For this review, take the finished solid that the model builds, in its own axes (mm). A direction names the side the tool comes from. Give positions to 0.01 mm unless a question says otherwise; leave off trailing zeros. Loops run counter-clockwise (first coordinate to the right, second up) from the corner with the lowest first, then second, coordinate; pieces in that order, holes last. Notation, with made-up numbers: (40, 42) -> (70, 42) arc R17 cw to (70, 52) -> close; hole circle Ø11 at (67, 4.25). An arc over 180 degrees is marked (long way). One line per question, with ' | ' between items. Start each with the question number.
(1) Tool access review of faces 5 (the flat face through (144, 5, 46)), 6 (the flat face through (-2, 30, 50)), 7 (the flat face through (155, 15, -46)): name each direction out of +Z, -Z, +X, -X, +Y, -Y from which nothing blocks a thin tool from reaching the whole face with its end or side.
(2) Insertion check: P1, Ø7.5, axis at x = 152.01, y = 7.99, coming from the +Z side; P2, Ø1, axis at x = 38, z = -35, coming from the +Y side; P3, Ø1.1, axis at x = 148.5, z = 7, coming from the +Y side. Each pin has a flat end and moves straight along its axis. Give the tip position at first contact, or say it passes through.
(3) Wall thickness on probe 1 along X at (y, z) = (19, 9); probe 2 along Z at (x, y) = (-105, 35.5); probe 3 along Y at (x, z) = (64, -24): over which ranges is each line inside the solid? List them lowest first.
(4) Consider section B-B (y = 18). Write out the cut boundary in (x, z).
(5) Consider section A-A (x = -73.5). Write out the cut boundary in (y, z), and give its area (3 significant figures).
(6) Draft analysis for pull direction Y (two halves, no side actions). For faces 1 (the flat face through (2, 0, 1)), 2 (the flat face through (2, 10, 1)), 3 (the cylindrical face through (155.18, 8.13, -54.07)), 4 (the flat face through (152, 4, -49)), state which applies: +Y half, -Y half, draft (parallel to the pull), parting line (faces both ways), or undercut.
Autodesk Inventor part; units mm, degrees
ref_plane "Work Plane1" through (-150, 50, -42.2) normal (0, 0, 1) x (1, 0, 0)
ref_plane "YZ Plane" through (0, 0, 0) normal (1, 0, 0) x (0, 1, 0)
ref_plane "XZ Plane" through (0, 0, 0) normal (0, 1, 0) x (-1, 0, 0)
sketch "Sketch1" plane through (0, 0, 0) normal (0, 1, 0) x (-1, 0, 0)
  line L0 (150, 50) -> (-150, 50)
  line L1 (-150, 50) -> (-150, -50)
  line L2 (-150, -50) -> (150, -50)
  line L3 (150, -50) -> (150, 50)
  line L4 (150, 50) -> (-150, -50) construction
  line L5 (-150, 50) -> (150, -50) construction
  line L6 (160, 60) -> (-160, 60)
  line L7 (-160, 60) -> (-160, -60)
  line L8 (-160, -60) -> (160, -60)
  line L9 (160, -60) -> (160, 60)
  point P0 (0, 0)
  dimension "d0" = 100
  dimension "d1" = 300
  dimension "d2" = 10
extrude "Extrusion1" add sketch "Sketch1" along normal blind 10 contours L3 L2 L1 L0
extrude "Extrusion2" add sketch "Sketch1" along normal blind 50
sketch "Sketch2" plane through (160, 0, -60) normal (0, 0, -1) x (-1, 0, 0)
  line L0 (0, 0) -> (0, 50)
  line L1 (0, 0) -> (0, 3.5)
  line L2 (0, 3.5) -> (3.5, 3.5)
  line L3 (3.5, 3.5) -> (7.9901, 7.9901)
  circle A0 centre (7.9901, 7.9901) radius 3.175
  point P0 (160, 0)
  dimension "d7" = 3.5
  dimension "d8" = 3.5
  dimension "d9" = 6.35
  dimension "d10" = 135
  dimension "d11" = 6.35
extrude "Extrusion3" cut sketch "Sketch2" against normal blind 150
fillet "Fillet1" radius 1 2 edges at (155.1849, 7.9901, -60) (155.1849, 7.9901, 60)
sketch "Sketch3" plane through (160, 0, 60) normal (1, 0, 0) x (0, 0, -1)
  line L0 (0, 0) -> (0, 50)
  line L1 (0, 0) -> (11, 0)
  line L2 (120, 0) -> (0, 0)
  line L3 (11, 0) -> (17.8, 0)
  line L4 (17.8, 0) -> (17.8, 15)
  line L5 (17.8, 15) -> (11, 15)
  line L6 (11, 15) -> (11, 0)
  line L7 (120, 0) -> (120, 50)
  line L8 (120, 0) -> (109, 0)
  line L9 (109, 0) -> (102.2, 0)
  line L10 (102.2, 0) -> (102.2, 15)
  line L11 (102.2, 15) -> (109, 15)
  line L12 (109, 15) -> (109, 0)
  point P0 (60, 0)
  point P1 (17.8, 0)
  dimension "d15" = 11
  dimension "d16" = 6.8
  dimension "d17" = 15
  dimension "d18" = 11
  dimension "d19" = 6.8
extrude "Extrusion4" cut sketch "Sketch3" against normal blind 13
ref_plane "Work Plane1" through (-150, 50, -42.2) normal (0, 0, 1) x (1, 0, 0)
sketch "Sketch4" plane through (-150, 50, -42.2) normal (0, 0, 1) x (1, 0, 0)
  circle A0 centre (302.0099, -42.0099) radius 4.175
  line L0 (300, -38.3505) -> (300, -37.0005)
  line L1 (300, -39.552) -> (300, 0)
  line L2 (297, -50) -> (297, -40)
  arc A1 (300, -37.0005) -> (297, -40) centre (299.8581, -39.8585) ccw
  line L3 (297, -40) -> (297.4, -40)
  line L4 (299.552, -40) -> (0, -40)
  line L5 (300, -37.0005) -> (300, -37.4005)
  arc A2 (300, -37.4005) -> (297.4, -40) centre (300.0042, -40.0047) ccw
  point P0 (150, -50)
  dimension "d23" = 1.35
  dimension "d24" = 0.4
  dimension "d25" = 0.4
extrude "Extrusion5" add sketch "Sketch4" along normal blind 84.4 contours A2 L3 A1 L0
sketch "Sketch5" plane through (0, 10, 0) normal (0, 1, 0) x (1, 0, 0)
  line L0 (147, 49) -> (147, 42.2)
  line L1 (147, 49) -> (144, 49)
  line L2 (144, 49) -> (144, 42.2)
  line L3 (144, 42.2) -> (147, 42.2)
  line L4 (147, 42.2) -> (147, 49)
  point P0 (0, 0)
  dimension "d28" = 3
extrude "Extrusion6" cut sketch "Sketch5" against normal blind 84.4
sketch "Sketch6" plane through (0, 10, 0) normal (0, 1, 0) x (1, 0, 0)
  line L0 (147, -49) -> (147, -42.2)
  line L1 (147, -49) -> (144, -49)
  line L2 (144, -49) -> (144, -42.2)
  line L3 (144, -42.2) -> (147, -42.2)
  line L4 (147, -42.2) -> (147, -49)
  point P0 (0, 0)
  dimension "d31" = 3
extrude "Extrusion7" cut sketch "Sketch6" against normal blind 84.4
properties part number "GiveBox"
A:
1) face 5: +X, +Y, -Y | face 6: +Y | face 7: +X, -Y
2) P1: stops at z = 59.91 | P2: stops at y = 10 | P3: stops at y = 12.89
3) probe 1: x = -160 to -150, 150 to 160 | probe 2: z = -60 to -50, 50 to 60 | probe 3: y = 0 to 10
4) outline: (-160, -60) -> (160, -60) -> (160, 60) -> (-160, 60) -> close; hole (-150, -50) -> (150, -50) -> (150, 50) -> (-150, 50) -> close
5) outline: (0, -60) -> (50, -60) -> (50, -50) -> (10, -50) -> (10, 50) -> (50, 50) -> (50, 60) -> (0, 60) -> close | area: 2,000 mm^2
6) face 1: -Y half | face 2: +Y half | face 3: undercut | face 4: draft
